Autodesk Inventor part; units mm, degrees
ref_plane "YZ Plane" through (0, 0, 0) normal (1, 0, 0) x (0, 1, 0)
ref_plane "XZ Plane" through (0, 0, 0) normal (0, 1, 0) x (-1, 0, 0)
ref_plane "XY Plane" through (0, 0, 0) normal (0, 0, 1) x (1, 0, 0)
sketch "Sketch1" plane through (0, 0, 0) normal (0, 1, 0) x (-1, 0, 0)
  circle A0 centre (29.6155, 33.147) radius 6.35 construction
  circle A1 centre (0, 0) radius 38.1 construction
  circle A2 centre (29.6155, -33.147) radius 6.35 construction
  circle A3 centre (29.6155, 33.147) radius 29.972 construction
  circle A4 centre (29.6155, -33.147) radius 29.972 construction
  line L0 (29.6155, 3.175) -> (29.6155, -3.175) construction
  circle A5 centre (0, 0) radius 40.64 construction
  circle A6 centre (-8.3197, 52.6872) radius 6.35 construction
  circle A7 centre (-8.3197, 52.6872) radius 3.2639
  line L1 (-7.3293, 46.4149) -> (-6.3388, 40.1426) construction
  line L2 (-2.6746, 49.7794) -> (2.9705, 46.8716) construction
  circle A8 centre (-8.3197, -52.6872) radius 6.35 construction
  circle A9 centre (-8.3197, -52.6872) radius 3.2639
  line L3 (-7.3293, -46.4149) -> (-6.3388, -40.1426) construction
  line L4 (2.9705, -46.8716) -> (-2.6746, -49.7794) construction
  circle A10 centre (56.4888, 0) radius 6.35 construction
  circle A11 centre (56.4888, 0) radius 3.2639
  line L5 (48.4908, 9.8652) -> (52.4898, 4.9326) construction
  line L6 (52.4898, -4.9326) -> (48.4908, -9.8652) construction
  circle A12 centre (0, 0) radius 14.2875
  circle A13 centre (29.6155, 33.147) radius 9.525
  circle A14 centre (29.6155, -33.147) radius 9.525
  circle A15 centre (29.6155, 33.147) radius 25.4 construction
  circle A16 centre (29.6155, 58.547) radius 2.794
  circle A17 centre (49.474, 48.9836) radius 2.794
  circle A18 centre (54.3787, 27.495) radius 2.794 construction
  circle A19 centre (40.6362, 10.2624) radius 2.794
  circle A20 centre (18.5949, 10.2624) radius 2.794
  circle A21 centre (4.8523, 27.495) radius 2.794
  circle A22 centre (9.757, 48.9836) radius 2.794
  circle A23 centre (29.6155, -33.147) radius 25.4 construction
  circle A24 centre (29.6155, -58.547) radius 2.794
  circle A25 centre (49.474, -48.9836) radius 2.794
  circle A26 centre (54.3787, -27.495) radius 2.794 construction
  circle A27 centre (40.6362, -10.2624) radius 2.794
  circle A28 centre (18.5949, -10.2624) radius 2.794
  circle A29 centre (4.8523, -27.495) radius 2.794
  circle A30 centre (9.757, -48.9836) radius 2.794
  line L7 (26.2955, 62.9346) -> (-9.0231, 58.9981)
  line L8 (-13.7609, 55.9607) -> (-34.8236, 20.9505)
  line L9 (-34.8236, -20.9505) -> (-13.7609, -55.9607)
  line L10 (-9.0231, -58.9981) -> (26.2955, -62.9346)
  line L11 (59.4535, -35.9782) -> (62.8105, -0.5998)
  line L12 (62.8105, 0.5998) -> (59.4535, 35.9782)
  arc A31 (-9.0231, 58.9981) -> (-13.7609, 55.9607) centre (-8.3197, 52.6872) ccw
  arc A32 (59.4535, 35.9782) -> (26.2955, 62.9346) centre (29.6155, 33.147) ccw
  arc A33 (-34.8236, 20.9505) -> (-34.8236, -20.9505) centre (0, 0) ccw
  arc A34 (-13.7609, -55.9607) -> (-9.0231, -58.9981) centre (-8.3197, -52.6872) ccw
  arc A35 (26.2955, -62.9346) -> (59.4535, -35.9782) centre (29.6155, -33.147) ccw
  arc A36 (62.8105, -0.5998) -> (62.8105, 0.5998) centre (56.4888, 0) ccw
  point P0 (29.6155, 0)
  dimension "d21" = 50.8
  dimension "d27" = 50.8
  dimension "d0" = 12.7
  dimension "d1" = 76.2
  dimension "d2" = 12.7
  dimension "d3" = 59.944
  dimension "d4" = 59.944
  dimension "d5" = 6.35
  dimension "d6" = 2.54
  dimension "d8" = 12.7
  dimension "d9" = 6.5278
  dimension "d11" = 6.35
  dimension "d12" = 12.7
  dimension "d13" = 6.5278
  dimension "d14" = 6.35
  dimension "d15" = 12.7
  dimension "d16" = 6.5278
  dimension "d17" = 6.35
  dimension "d18" = 6.35
  dimension "d19" = 28.575
  dimension "d20" = 19.05
  dimension "d22" = 5.588
  dimension "d25" = 360
  dimension "d30" = 360
extrude "Extrusion1" add sketch "Sketch1" along normal blind 6.35
properties material "Aluminum 6061"
The model under review builds one solid part; all positions refer to its coordinate system, in mm. Round coordinates to 2 decimals unless told otherwise and drop trailing zeros. Loops run counter-clockwise (first coordinate to the right, second up) from the corner with the lowest first, then second, coordinate; pieces in that order, holes last. Notation, with made-up numbers: M 70.5,47.25 L 109.5,47.25 A7 cw 109.5,59.25 Z; hole C 17,-1 d9. An arc over 180 degrees is marked long. Answer as a JSON object with one key per item and string values.
(1) Take a section at C-C on y = 5.25. Count the separate pieces of the cut face and the enclosed holes in it, and give its area (3 significant figures).
Resolved:
{"separate pieces": "1", "enclosed holes": "18", "area": "8,970 mm²"}
(2) Clearance check with flat-ended pins moving along their axes: P1, Ø2, axis at x = -12, y = 5, coming from the -Z side; P2, Ø1, axis at y = 1, z = -27, coming from the +X side; P3, Ø2, axis at y = 1, z = 41, coming from the -X side. State where each tip first meets the part, or that it passes through.
Resolved:
{"P1": "z = -61.45", "P2": "x = 31.48", "P3": "x = -58.79"}
(3) To check wall thickness, follow line 1 along Z through (x, y) = (-49.5, 2); line 2 along X through (y, z) = (1.25, 0.5); line 3 along Z through (x, y) = (-49, 5.25). State the ranges of each line that lie inside material, in increasing order.
Resolved:
{"line 1": "-55.57 to -51.78, -46.19 to 46.19, 51.78 to 55.57", "line 2": "-62.82 to -59.71, -53.26 to -14.28, 14.28 to 40.64", "line 3": "-56.01 to -51.74, -46.23 to 46.23, 51.74 to 56.01"}
(4) Draft analysis for pull direction X (two halves, no side actions). For faces 1 (the flat face through (-61.11, 3.13, -18.54)), 2 (the cylindrical face through (-20.1, 3.1, -33.6)), 3 (the flat face through (24.145, 3.131, 38.701)), state which applies: released by +X, released by -X, zero draft, split by the parting line, or undercut.
Resolved:
{"face 1": "released by -X", "face 2": "undercut", "face 3": "released by +X"}
(5) Take a section at A-A on z = -54. Give the boundary of the cut face in (x, y).
Resolved:
{"outline": "M -51.14,0 L 5.33,0 L 5.33,6.35 L -51.14,6.35 Z; M 11.31,0 L 14.94,0 L 14.94,6.35 L 11.31,6.35 Z"}
(6) Take a section at B-B on x = -40.5. Give the boundary of the cut face in (y, z), and give its area (3 significant figures).
Resolved:
{"outline": "M 0,-61.07 L 6.35,-61.07 L 6.35,-13.05 L 0,-13.05 Z; M 0,-7.47 L 6.35,-7.47 L 6.35,7.47 L 0,7.47 Z; M 0,13.05 L 6.35,13.05 L 6.35,61.07 L 0,61.07 Z", "area": "705 mm²"}
(7) Take a section at D-D on x = 0. Give the boundary of the cut face in (y, z), and give its area (3 significant figures).
Resolved:
{"outline": "M 0,-60 L 6.35,-60 L 6.35,-14.29 L 0,-14.29 Z; M 0,14.29 L 6.35,14.29 L 6.35,60 L 0,60 Z", "area": "581 mm²"}
